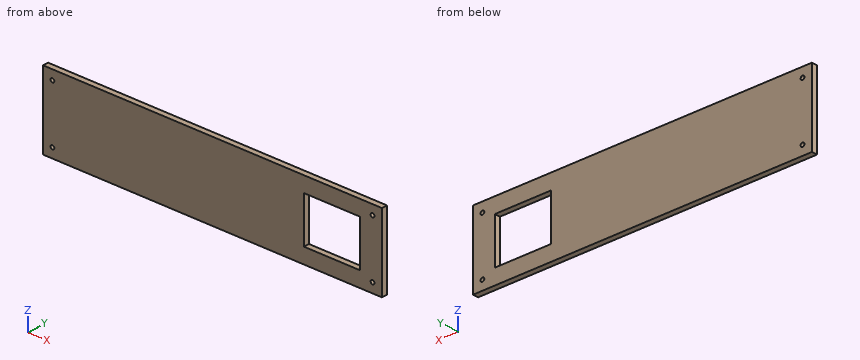
```python
from build123d import *

# Parameters (mm, degrees)
SKETCH1_W           = 900
SKETCH1_H           = 200
SKETCH1_W_2         = 149
SKETCH1_H_2         = 120
BOSS_EXTRUDE1_DEPTH = 15
SKETCH2_R           = 5
CUT_EXTRUDE1_DEPTH  = 462.221205063


with BuildPart() as part:
    # Sketch1 → Boss-Extrude1 (new body)
    with BuildSketch(Plane(origin=(0, 0, 0), x_dir=(1, 0, 0), z_dir=(0, 1, 0))):
        Rectangle(SKETCH1_W, SKETCH1_H)
        with Locations((317.5, 0)):
            Rectangle(SKETCH1_W_2, SKETCH1_H_2, mode=Mode.SUBTRACT)
    extrude(amount=BOSS_EXTRUDE1_DEPTH)

    # Sketch2 → Cut-Extrude1 (cut, through all)
    with BuildSketch(Plane(origin=(0, 0, 0), x_dir=(1, 0, 0), z_dir=(0, 1, 0))):
        with Locations(Location((-425, 75, 0), (0, 0, 270))):
            Circle(SKETCH2_R)
        with Locations(Location((-425, -75, 0), (0, 0, 90))):
            Circle(SKETCH2_R)
        with Locations(Location((425, 75, 0), (0, 0, 90))):
            Circle(SKETCH2_R)
        with Locations(Location((425, -75, 0), (0, 0, 270))):
            Circle(SKETCH2_R)
    extrude(amount=CUT_EXTRUDE1_DEPTH, mode=Mode.SUBTRACT)


solid = part.part
```
The listing builds one solid part. Answer for the finished solid, in the listing's coordinates (mm). Round coordinates to 2 decimals unless told otherwise and drop trailing zeros. Loops run counter-clockwise (first coordinate to the right, second up) from the corner with the lowest first, then second, coordinate; pieces in that order, holes last.
Q1. Find the intervals of material crossed by line 1 (Z direction, x = -425, y = 3.5); line 2 (X direction, y = 7.5, z = -75); line 3 (X direction, y = 4.75, z = -44), in increasing order.
Q2. Section B-B, the plane y = 10.75 is taken. Determine the outline of the cut face in (x, z).
Q3. Section A-A, the plane z = 42 is taken. Determine the outline of the cut face in (x, y), then the cut area to 3 significant figures.
Q4. Given pin 1 Ø5 at (x, z) = (-45, 22.5) entering from -Y, flat-ended and moving along its own axis, determine where the tip first touches the part or whether it passes through.
Q5. Section C-C, the plane x = 287.5 is taken. Determine the outline of the cut face in (y, z).
Completed:
1. line 1: z = -100 to -80, -70 to 70, 80 to 100
1. line 2: x = -450 to -430, -420 to 420, 430 to 450
1. line 3: x = -450 to 243, 392 to 450
2. outline: (-450, -100) - (450, -100) - (450, 100) - (-450, 100) - close; hole circle Ø10 at (-425, -75); hole circle Ø10 at (-425, 75); hole (243, -60) - (392, -60) - (392, 60) - (243, 60) - close; hole circle Ø10 at (425, -75); hole circle Ø10 at (425, 75)
3. outline: (-450, 0) - (243, 0) - (243, 15) - (-450, 15) - close; (392, 0) - (450, 0) - (450, 15) - (392, 15) - close
3. area: 11,300 mm2
4. pin 1: stops at y = 0
5. outline: (0, -100) - (15, -100) - (15, -60) - (0, -60) - close; (0, 60) - (15, 60) - (15, 100) - (0, 100) - close
